Can you work these out from the drawing? Everything is in mm from the part's minimum corner. A direction names the side the tool comes from. Coordinates: 2 decimals unless noted, no trailing zeros. Loops run counter-clockwise (first coordinate to the right, second up) from the corner with the lowest first, then second, coordinate; pieces in that order, holes last.
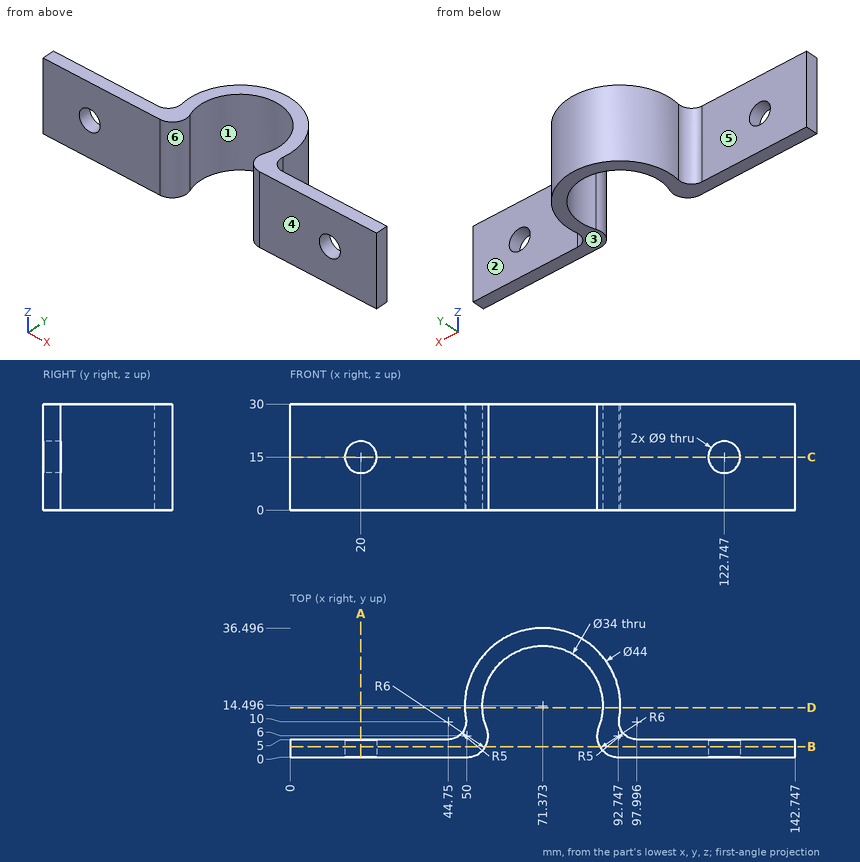
Item 1: Suppose I cut it at B-B, the plane y = 3. Please give me the cut outline in (x, z).
Results are:
outline: (0, 0) - (55.2, 0) - (55.2, 30) - (0, 30) - close; (87.55, 0) - (142.75, 0) - (142.75, 30) - (87.55, 30) - close; hole circle Ø9 at (20, 15); hole circle Ø9 at (122.75, 15)
Item 2: Suppose I cut it at C-C, the plane z = 15. Count the separate pieces of the cut face and the enclosed holes in it.
Results are:
separate pieces: 3
enclosed holes: 0
Item 3: I'm going to push flat-ended pins straight in: P1, Ø15, axis at x = 13.5, z = 19.5, coming from the +Y side; P2, Ø10, axis at y = 14, z = 13.5, coming from the -X side; P3, Ø4, axis at y = 24, z = 20.5, coming from the -X side. Where does each tip first touch, or does it pass through?
Results are:
P1: stops at y = 5
P2: stops at x = 49.37
P3: stops at x = 50.69
Item 4: On a 3-axis mill with a long thin cutter (end or side, diameter ignored), from which of +Z, -Z, +X, -X, +Y, -Y can I reach the whole of each face in a straight line? I mean the marked faces 1 and 2. Say none if no direction works.
Results are:
face 1: +Z, -Z
face 2: +Z, -Z, +X, +Y
Item 5: Suppose I cut it at A-A, the plane x = 20. Please give me the cut outline in (y, z), plus the area to 3 significant figures.
Results are:
outline: (0, 0) - (5, 0) - (5, 10.5) - (0, 10.5) - close; (0, 19.5) - (5, 19.5) - (5, 30) - (0, 30) - close
area: 105 mm2
Item 6: Suppose I cut it at D-D, the plane y = 14. Please give me the cut outline in (x, z), plus the area to 3 significant figures.
Results are:
outline: (49.38, 0) - (54.38, 0) - (54.38, 30) - (49.38, 30) - close; (88.37, 0) - (93.37, 0) - (93.37, 30) - (88.37, 30) - close
area: 300 mm2
Item 7: I need wall thicknesses on line 1 along X through (y, z) = (15, 22.5) (1 decimal); line 2 along Z through (x, y) = (20, 2); line 3 along Y through (x, z) = (133, 15). Which ranges of each line are inside material? Lowest first, please.
Results are:
line 1: x = 49.4 to 54.4, 88.4 to 93.4
line 2: z = 0 to 10.5, 19.5 to 30
line 3: y = 0 to 5
Item 8: We'd pull the mould along Y, two halves only. Please class the marked faces 3, 4, 5 and 6: +Y half, -Y half, draft (parallel to the pull), parting line (faces both ways), or undercut.
Results are:
face 3: draft
face 4: -Y half
face 5: +Y half
face 6: undercut
